from build123d import *

# Parameters (mm, degrees)
CUT_EXTRUDE1_DEPTH = 0.65
FILLET1_R          = 0.1
CHAMFER1_SIZE      = 0.2


with BuildPart() as part:
    # Sketch2 → Revolve1 (revolve)
    with BuildSketch(Plane(origin=(0, 0, 0), x_dir=(0, 0, -1), z_dir=(1, 0, 0)), mode=Mode.PRIVATE) as revolve1_sk:
        Polygon((-1.3, 0), (-1.3, 2.5), (0, 2.5), (0, 1.25), (10, 1.25), (10, 0), align=None)
    revolve(revolve1_sk.sketch.rotate(Axis((0, 0, 1.3), (0, 0, -1)), 90), axis=Axis((0, 0, 1.3), (0, 0, -1)))

    # Sketch3 → Cut-Extrude1 (cut)
    with BuildSketch(Plane.XY.offset(1.3)):
        Polygon((0, 0.72), (-0.623538291, 0.36), (-0.623538291, -0.36), (0, -0.72), (0.623538291, -0.36), (0.623538291, 0.36), align=None)
    extrude(amount=-CUT_EXTRUDE1_DEPTH, mode=Mode.SUBTRACT)

    # Fillet1
    fillet1_edges = [part.edges().sort_by_distance(p)[0] for p in [
        (-2.5, 0, 0),
        (-2.5, 0, 1.3),
    ]]
    fillet(fillet1_edges, radius=FILLET1_R)

    # Chamfer1
    chamfer1_edges = [part.edges().sort_by_distance(p)[0] for p in [
        (-1.25, 0, -10),
    ]]
    chamfer(chamfer1_edges, length=CHAMFER1_SIZE)

    # Sketch4 → Cut-Revolve1 (revolve, cut)
    with BuildSketch(Plane(origin=(0, 0, 0), x_dir=(0, 0, -1), z_dir=(1, 0, 0)), mode=Mode.PRIVATE) as cut_revolve1_sk:
        Polygon((-0.65, 0.72), (-0.217380354, 0), (-0.65, 0), align=None)
        Polygon((-1.3, 0.72), (-1.3, 0.57), (-1.21339746, 0.57), align=None)
    revolve(cut_revolve1_sk.sketch.rotate(Axis((0, 0, 0), (0, 0, -1)), 270), axis=Axis((0, 0, 0), (0, 0, -1)), mode=Mode.SUBTRACT)


solid = part.part
Verification items for the finished model (mm, model axes). A direction names the side the tool comes from. Round coordinates to 2 decimals unless told otherwise and drop trailing zeros. Order: outer loops, then holes, each group sorted by start corner. A loop starts at its lowest first (then second) coordinate and runs counter-clockwise, first axis right, second up.
1. Release check for a two-part mould opening along Y. For faces 3 (the cylindrical face through (-2.5, -0.1, 0.6)), 4 (the conical face through (0.025, -0.112, 0.286)), 5 (the flat face through (0, -1, 1.3)) record: +Y half, -Y half, draft (parallel to the pull), parting line (faces both ways), or undercut.
Final values:
face 3: parting line
face 4: undercut
face 5: draft
2. Section check B-B on z = 0.5. Record the cut outline in (x, y).
Final values:
outline: circle Ø5 at (0, 0); hole circle Ø0.94 at (0, 0)
3. Thickness scan on L1, parallel to Z at x = -1.4, y = 1; L2, parallel to X at y = -0.4, z = 1.25; L3, parallel to Y at x = -0.9, z = -8. Record the ranges inside material, lowest first.
Final values:
L1: z = 0 to 1.3
L2: x = -2.45 to -0.55, 0.55 to 2.45
L3: y = -0.87 to 0.87
4. Access from +Z, -Z, +X, -X, +Y, -Y to the whole of each face (thin tool, end or side, straight path). Record for faces 1 (the flat face through (1, 1, 0)), 2 (the flat face through (0, 0, -10)).
Final values:
face 1: -Z
face 2: -Z, +X, -X, +Y, -Y
5. Go/stop test with flat-tipped pins: P1, Ø2, axis at y = 0.5, z = -8.5, coming from the -X side; P2, Ø1, axis at x = -0.5, z = -5.5, coming from the -Y side. Record where each tip stops, or that it passes through.
Final values:
P1: stops at x = -1.25
P2: stops at y = -1.25
6. Section check A-A on z = -9.5. Record the cut outline in (x, y).
Final values:
outline: circle Ø2.5 at (0, 0)
